from build123d import *

# Parameters (mm, degrees)
SKETCH1_R           = 0.635
BOSS_EXTRUDE1_DEPTH = 5.08
SKETCH2_R           = 4.445
SKETCH2_R_2         = 0.635
BOSS_EXTRUDE2_DEPTH = 5.08
SKETCH3_R           = 3.2385
CUT_EXTRUDE1_DEPTH  = 6.35
FILLET1_R           = 0.254
FILLET2_R           = 2.54
FILLET3_R           = 1.27
SKETCH5_R           = 0.381
CUT_EXTRUDE3_DEPTH  = 83.603101422


with BuildPart() as part:
    # Sketch1 → Boss-Extrude1 (new body)
    with BuildSketch(Plane.XY):
        with BuildLine():
            Line((0, 0), (76.64958, 0))
            Line((76.64958, 0), (81.72958, 0))
            Line((81.72958, 0), (81.72958, 3.175))
            Line((81.72958, 3.175), (76.64958, 3.175))
            Line((76.64958, 3.175), (75.06208, 3.175))
            Line((75.06208, 3.175), (75.06208, 4.7625))
            ThreePointArc((75.06208, 4.7625), (70.29958, 9.525), (65.53708, 4.7625))
            Line((65.53708, 4.7625), (65.53708, 3.175))
            Line((65.53708, 3.175), (11.1125, 3.175))
            Line((11.1125, 3.175), (11.1125, 4.7625))
            ThreePointArc((11.1125, 4.7625), (6.35, 9.525), (1.5875, 4.7625))
            Line((1.5875, 4.7625), (1.5875, 3.175))
            Line((1.5875, 3.175), (0, 3.175))
            Line((0, 3.175), (-5.08, 3.175))
            Line((-5.08, 3.175), (-5.08, 0))
            Line((-5.08, 0), (0, 0))
        make_face()
        with Locations((6.35, 4.7625)):
            Circle(SKETCH1_R, mode=Mode.SUBTRACT)
        with Locations((70.29958, 4.7625)):
            Circle(SKETCH1_R, mode=Mode.SUBTRACT)
    extrude(amount=BOSS_EXTRUDE1_DEPTH)

    # Sketch2 → Boss-Extrude2 (add)
    # profile 1 of 2: a face of its own
    with BuildSketch(Plane.XY.offset(5.08)):
        with Locations((6.35, 4.7625)):
            Circle(SKETCH2_R)
        with Locations((6.35, 4.7625)):
            Circle(SKETCH2_R_2, mode=Mode.SUBTRACT)
    # profile 2 of 2: a face of its own
    with BuildSketch(Plane.XY.offset(5.08)):
        with Locations((70.29958, 4.7625)):
            Circle(SKETCH2_R)
        with Locations((70.29958, 4.7625)):
            Circle(SKETCH2_R_2, mode=Mode.SUBTRACT)
    extrude(amount=BOSS_EXTRUDE2_DEPTH)

    # Sketch3 → Cut-Extrude1 (cut)
    with BuildSketch(Plane.XY.offset(10.16)):
        with Locations((6.35, 4.7625)):
            Circle(SKETCH3_R)
        with Locations((70.29958, 4.7625)):
            Circle(SKETCH3_R)
    extrude(amount=-CUT_EXTRUDE1_DEPTH, mode=Mode.SUBTRACT)

    # Fillet1
    fillet1_edges = [part.edges().sort_by_distance(p)[0] for p in [
        (1.905, 4.7625, 5.08),
        (65.85458, 4.7625, 5.08),
    ]]
    fillet(fillet1_edges, radius=FILLET1_R)

    # Fillet2
    fillet2_edges = [part.edges().sort_by_distance(p)[0] for p in [
        (75.06208, 3.175, 2.54),
        (11.1125, 3.175, 2.54),
        (65.53708, 3.175, 2.54),
        (1.5875, 3.175, 2.54),
    ]]
    fillet(fillet2_edges, radius=FILLET2_R)

    # Fillet3
    fillet3_edges = [part.edges().sort_by_distance(p)[0] for p in [
        (-5.08, 3.175, 2.54),
        (81.72958, 3.175, 2.54),
    ]]
    fillet(fillet3_edges, radius=FILLET3_R)

    # Sketch5 → Cut-Extrude3 (cut, through all)
    with BuildSketch(Plane(origin=(0, 3.175, 0), x_dir=(1, 0, 0), z_dir=(0, 1, 0))):
        with Locations(Location((-2.413, -2.54, 0), (0, 0, 180))):
            Circle(SKETCH5_R)
        with Locations(Location((79.06258, -2.54, 0), (0, 0, 180))):
            Circle(SKETCH5_R)
        with Locations(Location((61.53658, -2.54, 0), (0, 0, 180))):
            Circle(SKETCH5_R)
        with Locations(Location((15.113, -2.54, 0), (0, 0, 180))):
            Circle(SKETCH5_R)
    extrude(amount=-CUT_EXTRUDE3_DEPTH, mode=Mode.SUBTRACT)


solid = part.part
Verification items for the finished model (mm, model axes). A direction names the side the tool comes from. Round coordinates to 2 decimals unless told otherwise and drop trailing zeros. Loops run counter-clockwise (first coordinate to the right, second up) from the corner with the lowest first, then second, coordinate; pieces in that order, holes last. Notation, with made-up numbers: (-11.5, 54) - (29.5, 54) arc R24 cw to (29.5, 67) - close; hole circle Ø2 at (32.25, 41). An arc over 180 degrees is marked (long way). Use one line per item in the form item = value.
1. Section check B-B on x = 25.5. Record the cut outline in (y, z) (3 decimals).
A:
outline = (0, 0) - (3.175, 0) - (3.175, 5.08) - (0, 5.08) - close
2. Access from +Z, -Z, +X, -X, +Y, -Y to the whole of each face (thin tool, end or side, straight path). Record for faces 1 (the flat face through (6, 4, 3.81)), 2 (the flat face through (-2, 3.175, 3)), 3 (the flat face through (79, 3.175, 2)).
A:
face_1 = +Z
face_2 = +Z, -Z, -X, +Y
face_3 = +Z, -Z, +X, +Y
3. Draft check along Y on faces 4 (the cylindrical face through (5.65, 1.6, 7.03)), 5 (the flat face through (70, 4, 3.81)), 6 (the flat face through (39, 3.175, 3)), 7 (the cylindrical face through (65.86, 4.96, 7.71)). Enter one of: pulls with the +Y half, pulls with the -Y half, needs draft (parallel to the pull), parting line crosses it, or undercut.
A:
face_4 = undercut
face_5 = undercut
face_6 = pulls with the +Y half
face_7 = parting line crosses it
4. Section check A-A on z = 6.5. Give the number of separate pieces and of enclosed holes in the cut face, and give its area (3 significant figures).
A:
separate_pieces = 2
enclosed_holes = 2
area = 58.2 mm²
5. Scan lines: probe 1 along Y at (x, z) = (6.35, 7.25); probe 2 along X at (y, z) = (1.5, 2.5); probe 3 along X at (y, z) = (4.25, 6.5). Record each from-to range of solid material in increasing order.
A:
probe_1 = 0.32 to 1.52, 8 to 9.21
probe_2 = -5.08 to -2.79, -2.03 to 14.73, 15.49 to 61.16, 61.92 to 78.68, 79.44 to 81.73
probe_3 = 1.93 to 3.15, 9.55 to 10.77, 65.88 to 67.1, 73.5 to 74.71
6. Gauge pin test, flat ends, axial feed: pin 1 Ø1.5 at (x, z) = (47.5, 2) entering from +Y (3 decimals); pin 2 Ø2 at (y, z) = (7, 6.5) entering from +X; pin 3 Ø3 at (y, z) = (8, 3.5) entering from -X. Record the tip position at first contact, or that the pin passes through.
A:
pin_1 = 3.175
pin_2 = 74.57
pin_3 = 1.92
